Geometry check sheet. Reference: the model listing, model coordinates, mm. Face numbers are marked on the shaded views. A direction names the side the tool comes from. Coordinates: 2 decimals unless noted, no trailing zeros. Order: outer loops, then holes, each group sorted by start corner. A loop starts at its lowest first (then second) coordinate and runs counter-clockwise, first axis right, second up. Notation, with made-up numbers: (-6, 69.5) - (30, 69.5) arc R28 cw to (30, 100.5) - close; hole circle Ø7 at (-34.75, 33). An arc over 180 degrees is marked (long way). Return JSON: item names as keys, results as strings. Group by question number.
Item 1: Draft check along Z on the marked faces 4, 5 and 6. Enter one of: pulls with the +Z half, pulls with the -Z half, needs draft (parallel to the pull), parting line crosses it, or undercut.
Item 2: Tool access check on the marked faces 1, 2 and 3. Record the directions out of +Z, -Z, +X, -X, +Y, -Y that give a thin tool (end or side, any length) a straight path to the whole face; none if there is none.
Item 3: Scan lines: probe 1 along Y at (x, z) = (0, 5.2) (3 decimals); probe 2 along X at (y, z) = (-6.25, 2.75); probe 3 along Y at (x, z) = (-4.25, 6.75). Record each from-to range of solid material in increasing order.
Item 4: Section check A-A on y = 0. Enter the section's corners in (x, z) (3 decimals), then the cut area to 3 significant figures.
Item 5: Section check D-D on z = 3. Enter the section's corners in (x, y) (3 decimals), then the cut area to 3 significant figures.
Item 6: Section check C-C on z = 9.5. Enter the section's corners in (x, y) (3 decimals), then the cut area to 3 significant figures.
Item 7: Gauge pin test, flat ends, axial feed: pin 1 (3 mm diameter, centred on x = 2.5, z = 4, fed in from -Y); pin 2 (10 mm diameter, centred on x = -4.5, y = 2.5, fed in from -Z); pin 3 (5 mm diameter, centred on y = -8.5, z = 5, fed in from +X). Record the tip position at first contact, or that the pin passes through.
Autodesk Inventor part; units mm, degrees
ref_plane "YZ Plane" through (0, 0, 0) normal (1, 0, 0) x (0, 1, 0)
ref_plane "XZ Plane" through (0, 0, 0) normal (0, 1, 0) x (-1, 0, 0)
ref_plane "XY Plane" through (0, 0, 0) normal (0, 0, 1) x (1, 0, 0)
sketch "Sketch1" plane through (0, 0, 0) normal (0, 0, 1) x (1, 0, 0)
  circle A0 centre (0, 0) radius 12.195
  dimension "d0" = 24.39
extrude "Extrusion1" add sketch "Sketch1" along normal blind 10.23
sketch "Sketch2" plane through (0, 0, 0) normal (1, 0, 0) x (0, 1, 0)
  line L0 (-12.195, 0) -> (-12.195, 10.23)
  line L1 (9.375, 5.115) -> (9.375, 5.39)
  line L2 (9.375, 5.39) -> (9.375, 4.84)
  line L3 (9.375, 4.84) -> (9.375, 5.39)
  line L4 (12.195, 7.81) -> (9.775, 5.39)
  line L5 (12.195, 7.81) -> (15.6174, 7.81) construction
  line L6 (12.195, 7.81) -> (9.775, 10.23)
  line L7 (9.775, 4.84) -> (12.195, 2.42)
  line L8 (12.195, 2.42) -> (9.775, 0)
  line L9 (9.775, 4.84) -> (9.375, 4.84)
  line L10 (9.375, 5.39) -> (9.775, 5.39)
  line L11 (12.195, 7.81) -> (9.775, 10.23)
  line L12 (9.775, 10.23) -> (13.6006, 10.23)
  line L13 (13.6006, 10.23) -> (13.6006, 0)
  line L14 (13.6006, 0) -> (9.775, 0)
  line L15 (-12.195, 0) -> (12.195, 0)
  line L16 (0, -2.046) -> (0, 12.276)
  point P0 (0, 0)
  dimension "d4" = 0.275
  dimension "d5" = 0.55
  dimension "d6" = 135
revolve "Revolution1" cut sketch "Sketch2" angle 360 about axis through (0, 0, -10) along (0, 0, 1)
sketch "Sketch3" plane through (0, 0, 0) normal (0, 0, -1) x (-1, 0, 0)
  circle A0 centre (0, 0) radius 9.775
  circle A1 centre (0, 0) radius 6.945
  dimension "d8" = 13.89
extrude "Extrusion2" cut sketch "Sketch3" against normal blind 30 contours A1
sketch "Sketch4" plane through (0, 0, 0) normal (0, 0, -1) x (-1, 0, 0)
  circle A0 centre (0, 0) radius 7.987
  dimension "d11" = 15.974
extrude "Extrusion3" cut sketch "Sketch4" against normal blind 4.615
sketch "Sketch5" plane through (0, 0, 10.23) normal (0, 0, 1) x (1, 0, 0)
  circle A0 centre (0, 0) radius 7.987
  dimension "d14" = 15.974
extrude "Extrusion4" cut sketch "Sketch5" against normal blind 4.615
properties part number "dELRIN"
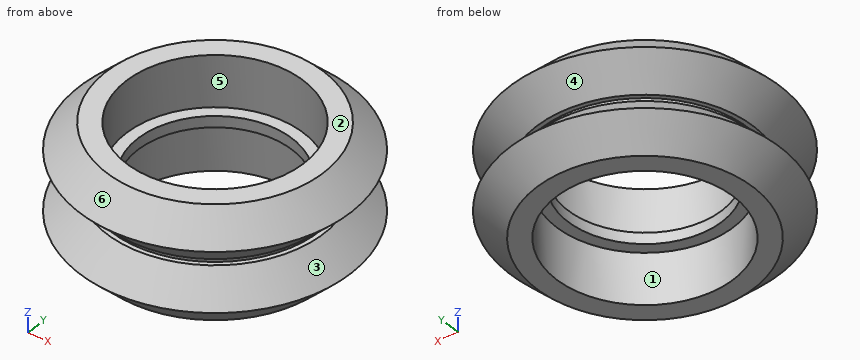
Computed:
{
 "1": {"face 4": "undercut", "face 5": "needs draft", "face 6": "pulls with the +Z half"},
 "2": {"face 1": "-Z", "face 2": "+Z, +X, -X, +Y, -Y", "face 3": "none"},
 "3": {"probe 1": "y = -9.375 to -6.945, 6.945 to 9.375", "probe 2": "x = -10.09 to -4.97, 4.97 to 10.09", "probe 3": "y = -10.29 to -6.76, 6.76 to 10.29"},
 "4": {"outline": "(-12.195, 2.42) - (-9.775, 0) - (-7.987, 0) - (-7.987, 4.615) - (-6.945, 4.615) - (-6.945, 5.615) - (-7.987, 5.615) - (-7.987, 10.23) - (-9.775, 10.23) - (-12.195, 7.81) - (-9.775, 5.39) - (-9.375, 5.39) - (-9.375, 4.84) - (-9.775, 4.84) - close; (6.945, 4.615) - (7.987, 4.615) - (7.987, 0) - (9.775, 0) - (12.195, 2.42) - (9.775, 4.84) - (9.375, 4.84) - (9.375, 5.39) - (9.775, 5.39) - (12.195, 7.81) - (9.775, 10.23) - (7.987, 10.23) - (7.987, 5.615) - (6.945, 5.615) - close", "area": "61.7 mm²"},
 "5": {"outline": "circle Ø23.23 at (0, 0); hole circle Ø15.974 at (0, 0)", "area": "223 mm²"},
 "6": {"outline": "circle Ø21.01 at (0, 0); hole circle Ø15.974 at (0, 0)", "area": "146 mm²"},
 "7": {"pin 1": "stops at y = -11.88", "pin 2": "stops at z = 0", "pin 3": "stops at x = 9.29"}
}
